Read the model definition and answer for the solid it produces. Units are mm, in the model's axes. A direction names the side the tool comes from. Give positions to 0.01 mm unless a question says otherwise; leave off trailing zeros. Order: outer loops, then holes, each group sorted by start corner. A loop starts at its lowest first (then second) coordinate and runs counter-clockwise, first axis right, second up.
Solid Edge part; units mm, degrees
sketch "Sketch1" plane through (0, 0, 0) normal (0, -1, 0) x (1, 0, 0)
  line L0 (-5.1, 8) -> (-5.1, 12.05)
  line L1 (-5.1, 12.05) -> (5.1, 12.05)
  line L2 (5.1, 12.05) -> (5.1, 8)
  line L3 (5.1, 8) -> (5.4, 8)
  line L4 (5.4, 8) -> (5.4, 2.5)
  line L5 (-5.4, 2.5) -> (5.4, 2.5)
  line L6 (-5.4, 8) -> (-5.4, 2.5)
  line L7 (-5.1, 8) -> (-5.4, 8)
  dimension "D1" = 5.1
revolve "RevolvedProtrusion1" add sketch "Sketch1" angle 360 about axis through (0, 0, 0) along (1, 0, 0)
chamfer "Chamfer1" distance 2 angle 45 2 edges at (-5.1, 0, -12.05) (5.1, 0, -12.05)
1) The part is cut by section D-D on x = 1. Determine the outline of the cut face in (y, z).
Final values:
outline: circle Ø24.1 at (0, 0); hole circle Ø5 at (0, 0)
2) The part is cut by section A-A on y = 0. Determine the outline of the cut face in (x, z), and give its area (3 significant figures).
Final values:
outline: (-5.4, -8) - (-5.1, -8) - (-5.1, -10.05) - (-3.1, -12.05) - (3.1, -12.05) - (5.1, -10.05) - (5.1, -8) - (5.4, -8) - (5.4, -2.5) - (-5.4, -2.5) - close; (-5.4, 2.5) - (5.4, 2.5) - (5.4, 8) - (5.1, 8) - (5.1, 10.05) - (3.1, 12.05) - (-3.1, 12.05) - (-5.1, 10.05) - (-5.1, 8) - (-5.4, 8) - close
area: 193 mm2
3) A tool of negligible diameter and unlimited length cuts with its end or side. For faces 4 (the face through (-5.25, -7.81, -1.73)), 5 (the face through (5.1, 8.14, -0.79)), 6 (the face through (0.043, -8.144, -8.881)), from which of +Z, -Z, +X, -X, +Y, -Y can it reach the whole face along a straight path? Write none if from no direction.
Final values:
face 4: -X
face 5: +X
face 6: +X, -X
4) The part is cut by section C-C on x = -3.75. Determine the outline of the cut face in (y, z), and give its area (3 significant figures).
Final values:
outline: circle Ø22.8 at (0, 0); hole circle Ø5 at (0, 0)
area: 389 mm2
5) Given pin 1 (1 mm diameter, centred on x = 4, z = -9.5, fed in from -Y); pin 2 (1 mm diameter, centred on x = -0.5, y = -7, fed in from -Z); pin 3 (6 mm diameter, centred on x = -4, z = -9.5, fed in from +Y), each flat-ended and moving along its own axis, determine where each tip first touches the part or whether it passes through.
Final values:
pin 1: stops at y = -6.98
pin 2: stops at z = -10.15
pin 3: stops at y = 10.06
6) For a pull along Z with two mould halves and no side action, classify faces 1 (the face through (0.08, 2.44, -0.54)), 2 (the face through (5.25, 7.81, -1.73)), 3 (the face through (-5.4, 2, -2)) as released by +Z, released by -Z, zero draft, split by the parting line, or undercut.
Final values:
face 1: undercut
face 2: split by the parting line
face 3: zero draft
7) Consider L1, parallel to Y at x = -1.5, z = 0; L2, parallel to X at y = 4.5, z = 8.5. Determine where each line is inside the solid, lowest interval first.
Final values:
L1: y = -12.05 to -2.5, 2.5 to 12.05
L2: x = -5.1 to 5.1
